Verification items for the finished model (mm, model axes). A direction names the side the tool comes from. Round coordinates to 2 decimals unless told otherwise and drop trailing zeros. Order: outer loops, then holes, each group sorted by start corner. A loop starts at its lowest first (then second) coordinate and runs counter-clockwise, first axis right, second up. Notation, with made-up numbers: M 67,21.25 L 118,21.25 A31 ccw 118,60.25 Z; hole C 16.5,29 d11. An arc over 180 degrees is marked long. Use CSV: the item, a comma, the result in double quotes. Start each with the question number.
Q1. Sectioned sample at B-B (y = 1.85). Enter the section's corners in (x, z) (3 decimals), and give its area (3 significant figures).
Q2. Sectioned sample at D-D (z = -5.5). Enter the section's corners in (x, y) (3 decimals), and give its area (3 significant figures).
Q3. Sectioned sample at A-A (z = 0). Enter the section's corners in (x, y) (3 decimals), and give its area (3 significant figures).
Q4. Mould release check, pull along X, two halves, no side actions. Record for faces 1 (the face through (16, 0, 0)), 2 (the face through (-10, 2, -3.175)): +X half, -X half, draft (parallel to the pull), parting line (faces both ways), or undercut.
Q5. Sectioned sample at C-C (x = 0.5). Enter the section's corners in (y, z) (3 decimals), and give its area (3 significant figures).
Q6. Set-up check for faces 3 (the face through (59.8, 1.57, -0.26)), 4 (the face through (-51, 2, -4)), 5 (the face through (33.6, 1.6, 4.5)): record each of +Z, -Z, +X, -X, +Y, -Y from which the full face is reachable in a straight line by a thin tool's end or side.
Q7. Scan lines: line 1 (X direction, y = 1.6, z = 0.5); line 2 (Z direction, x = -22, y = 0.85) (3 decimals); line 3 (Z direction, x = 38, y = 0.4). Record each from-to range of solid material in increasing order.
Q8. Gauge pin test, flat ends, axial feed: pin 1 Ø2.5 at (x, z) = (57.785, 0) entering from +Y; pin 2 Ø4.5 at (x, z) = (-57.785, 0) entering from +Y (3 decimals); pin 3 Ø1 at (x, y) = (-3, 2) entering from +Z (3 decimals). Record the tip position at first contact, or that the pin passes through.
```python
from build123d import *

# Parameters (mm, degrees)
SKETCH1_R           = 2.032
BOSS_EXTRUDE1_DEPTH = 3.175
FILLET2_DEPTH       = 3.175


with BuildPart() as part:
    # Sketch1 → Boss-Extrude1 (new body)
    with BuildSketch(Plane(origin=(0, 0, 0), x_dir=(1, 0, 0), z_dir=(0, 1, 0))):
        with BuildLine():
            Line((-38.735, -3.175), (38.735, -3.175))
            Line((38.735, -3.175), (55.045918919, -8.457513514))
            ThreePointArc((55.045918919, -8.457513514), (66.675, 0), (55.045918919, 8.457513514))
            Line((55.045918919, 8.457513514), (38.735, 3.175))
            Line((38.735, 3.175), (-38.735, 3.175))
            Line((-38.735, 3.175), (-57.486999924, 4.434999544))
            ThreePointArc((-57.486999924, 4.434999544), (-62.23, 0), (-57.486999924, -4.434999544))
            Line((-57.486999924, -4.434999544), (-38.735, -3.175))
        make_face()
        with Locations(Location((-57.785, 0, 0), (0, 0, 270))):
            Circle(SKETCH1_R, mode=Mode.SUBTRACT)
        with Locations(Location((57.785, 0, 0), (0, 0, 270))):
            Circle(SKETCH1_R, mode=Mode.SUBTRACT)
    extrude(amount=BOSS_EXTRUDE1_DEPTH)

    # Fillet2: read off the stored shape, not the designer's step
    # Fillet2 outline → Fillet2 (add)
    with BuildSketch(Plane(origin=(0, 0, 0), x_dir=(1, 0, 0), z_dir=(0, 1, 0))):
        with BuildLine():
            ThreePointArc((55.045918919, 8.457513514), (55.322751331, 8.542214672), (55.602194863, 8.617857143))
            ThreePointArc((55.602194863, 8.617857143), (33.943137383, 4.540961334), (11.946092127, 3.175))
            Line((11.946092127, 3.175), (38.735, 3.175))
            Line((38.735, 3.175), (55.045918919, 8.457513514))
        make_face()
        with BuildLine():
            ThreePointArc((-44.6882895, -3.575018243), (-38.731643046, -3.275032701), (-32.76828646, -3.175))
            Line((-32.76828646, -3.175), (-38.735, -3.175))
            Line((-38.735, -3.175), (-44.6882895, -3.575018243))
        make_face()
        with BuildLine():
            ThreePointArc((11.946092127, -3.175), (33.943137383, -4.540961334), (55.602194863, -8.617857143))
            ThreePointArc((55.602194863, -8.617857143), (55.322751331, -8.542214672), (55.045918919, -8.457513514))
            Line((55.045918919, -8.457513514), (38.735, -3.175))
            Line((38.735, -3.175), (11.946092127, -3.175))
        make_face()
        with BuildLine():
            Line((-38.735, 3.175), (-32.76828646, 3.175))
            ThreePointArc((-32.76828646, 3.175), (-38.731643046, 3.275032701), (-44.6882895, 3.575018243))
            Line((-44.6882895, 3.575018243), (-38.735, 3.175))
        make_face()
    extrude(amount=FILLET2_DEPTH)


solid = part.part
```
Verdict:
1,outline,"M -57.487,-4.435 L -44.688,-3.575 A177.8 cw -32.768,-3.175 L 11.946,-3.175 A177.8 cw 55.602,-8.618 A8.89 ccw long 55.602,8.618 A177.8 cw 11.946,3.175 L -32.768,3.175 A177.8 cw -44.688,3.575 L -57.487,4.435 A4.445 ccw long Z; hole C -57.785,0 d4.064; hole C 57.785,0 d4.064"
1,area,"1,070 mm²"
2,outline,"M 40.606,0 L 64.769,0 L 64.769,3.175 L 40.606,3.175 Z"
2,area,"76.7 mm²"
3,outline,"M -62.23,0 L -59.817,0 L -59.817,3.175 L -62.23,3.175 Z; M -55.753,0 L 55.753,0 L 55.753,3.175 L -55.753,3.175 Z; M 59.817,0 L 66.675,0 L 66.675,3.175 L 59.817,3.175 Z"
3,area,"383 mm²"
4,face 1,"draft"
4,face 2,"undercut"
5,outline,"M 0,-3.175 L 3.175,-3.175 L 3.175,3.175 L 0,3.175 Z"
5,area,"20.2 mm²"
6,face 3,"+Y, -Y"
6,face 4,"-Z, +Y, -Y"
6,face 5,"+Z, +Y, -Y"
7,line 1,"x = -62.2 to -59.75, -55.82 to 55.82, 59.75 to 66.66"
7,line 2,"z = -3.175 to 3.175"
7,line 3,"z = -5.09 to 5.09"
8,pin 1,"passes through"
8,pin 2,"stops at y = 3.175"
8,pin 3,"stops at z = 3.175"
